```python
from build123d import *

# Parameters (mm, degrees)
SKETCH1_W           = 100
SKETCH1_H           = 200
BOSS_EXTRUDE1_DEPTH = 2.5
SKETCH2_W           = 200
SKETCH2_H           = 70
BOSS_EXTRUDE2_DEPTH = 2.5
SKETCH3_R           = 8
CUT_EXTRUDE1_DEPTH  = 5
SKETCH4_W           = 105
SKETCH4_H           = 70
BOSS_EXTRUDE3_DEPTH = 10
SKETCH5_W           = 105
SKETCH5_H           = 70
BOSS_EXTRUDE4_DEPTH = 5
SKETCH6_W           = 100
SKETCH6_H           = 30
CUT_EXTRUDE2_DEPTH  = 167.37683132
SKETCH7_R           = 4
CUT_EXTRUDE5_DEPTH  = 232.381719243
SKETCH7_5_R         = 3
SKETCH7_5_R_2       = 8
CUT_EXTRUDE6_DEPTH  = 5
SKETCH8_R           = 8
CUT_EXTRUDE7_DEPTH  = 6
SKETCH9_W           = 105
SKETCH9_H           = 175
CUT_EXTRUDE8_DEPTH  = 15


with BuildPart() as part:
    # Sketch1 → Boss-Extrude1 (new, symmetric)
    with BuildSketch(Plane(origin=(0, 0, 0), x_dir=(1, 0, 0), z_dir=(0, 1, 0))):
        Rectangle(SKETCH1_W, SKETCH1_H)
    extrude(amount=BOSS_EXTRUDE1_DEPTH, both=True)

    # Sketch2 → Boss-Extrude2 (add, symmetric)
    with BuildSketch(Plane.ZY.offset(50)):
        with Locations((0, 32.5)):
            Rectangle(SKETCH2_W, SKETCH2_H)
    boss_extrude2 = extrude(amount=BOSS_EXTRUDE2_DEPTH, both=True)

    # Sketch3 → Cut-Extrude1 (cut)
    with BuildSketch(Plane.ZY.offset(52.5)):
        with Locations((-80, 25)):
            Circle(SKETCH3_R)
        with Locations((80, 25)):
            Circle(SKETCH3_R)
    cut_extrude1 = extrude(amount=-CUT_EXTRUDE1_DEPTH, mode=Mode.SUBTRACT)

    # Mirror1: Boss-Extrude2, Cut-Extrude1 across plane
    add(boss_extrude2.mirror(Plane(origin=(0, 0, 0), x_dir=(0, 0, 1), z_dir=(1, 0, 0))))
    add(cut_extrude1.mirror(Plane(origin=(0, 0, 0), x_dir=(0, 0, 1), z_dir=(1, 0, 0))), mode=Mode.SUBTRACT)

    # Sketch4 → Boss-Extrude3 (add)
    with BuildSketch(Plane(origin=(0, 0, -100), x_dir=(-1, 0, 0), z_dir=(0, 0, -1))):
        with Locations((0, 32.5)):
            Rectangle(SKETCH4_W, SKETCH4_H)
    extrude(amount=BOSS_EXTRUDE3_DEPTH)

    # Sketch5 → Boss-Extrude4 (add)
    with BuildSketch(Plane.XY.offset(100)):
        with Locations((0, 32.5)):
            Rectangle(SKETCH5_W, SKETCH5_H)
    extrude(amount=BOSS_EXTRUDE4_DEPTH)

    # Sketch6 → Cut-Extrude2 (cut, through all)
    with BuildSketch(Plane.ZY.offset(52.5)):
        with Locations((0, 25)):
            Rectangle(SKETCH6_W, SKETCH6_H)
    extrude(amount=-CUT_EXTRUDE2_DEPTH, mode=Mode.SUBTRACT)

    # Sketch7 → Cut-Extrude5 (cut, through all)
    with BuildSketch(Plane(origin=(0, 0, 105), x_dir=(-1, 0, 0), z_dir=(0, 0, -1))):
        with Locations(Location((35, 40.5, 0), (0, 0, 180))):
            Circle(SKETCH7_R)
        with Locations(Location((-35, 40.5, 0), (0, 0, 180))):
            Circle(SKETCH7_R)
    extrude(amount=CUT_EXTRUDE5_DEPTH, mode=Mode.SUBTRACT)

    # Sketch7<5> → Cut-Extrude6 (cut)
    with BuildSketch(Plane(origin=(0, 0, 105), x_dir=(-1, 0, 0), z_dir=(0, 0, -1))):
        with Locations(Location((15.5, 56, 0), (0, 0, 180))):
            Circle(SKETCH7_5_R)
        with Locations(Location((-15.5, 56, 0), (0, 0, 180))):
            Circle(SKETCH7_5_R)
        with Locations(Location((15.5, 25, 0), (0, 0, 180))):
            Circle(SKETCH7_5_R)
        with Locations(Location((-15.5, 25, 0), (0, 0, 180))):
            Circle(SKETCH7_5_R)
        with Locations(Location((0, 40.5, 0), (0, 0, 180))):
            Circle(SKETCH7_5_R_2)
    extrude(amount=CUT_EXTRUDE6_DEPTH, mode=Mode.SUBTRACT)

    # Sketch8 → Cut-Extrude7 (cut)
    with BuildSketch(Plane(origin=(0, 0, -100), x_dir=(-1, 0, 0), z_dir=(0, 0, -1))):
        with Locations(Location((0, 40.5, 0), (0, 0, 180))):
            Circle(SKETCH8_R)
    extrude(amount=CUT_EXTRUDE7_DEPTH, mode=Mode.SUBTRACT)

    # Sketch9 → Cut-Extrude8 (cut)
    with BuildSketch(Plane(origin=(0, 67.5, 0), x_dir=(1, 0, 0), z_dir=(0, 1, 0))):
        with Locations((0, 22.5)):
            Rectangle(SKETCH9_W, SKETCH9_H)
    extrude(amount=-CUT_EXTRUDE8_DEPTH, mode=Mode.SUBTRACT)


solid = part.part
```
Input: part model. Units: mm. Frame: model coordinates. A direction names the side the tool comes from. Round coordinates to 2 decimals unless told otherwise and drop trailing zeros. Write each loop counter-clockwise with the first axis right and the second up, starting at its lowest first coordinate (ties: lowest second). Pieces come first, ordered by that corner, then holes. Notation, with made-up numbers: (-38.75, 77) - (-15.75, 77) arc R26 cw to (-15.75, 96) - close; hole circle Ø6 at (-35, 69). An arc over 180 degrees is marked (long way). Write item = value, one per line.
(1) Pull-direction query (Y, two-part tool) for faces 6 (the flat face through (-1, -2.5, -4)), 7 (the flat face through (47.5, 43, -1)), 8 (the cylindrical face through (-50, 30.4, -85.9)); classes: +Y half, -Y half, draft (parallel to the pull), parting line (faces both ways), or undercut.
Geometry check:
face_6 = -Y half
face_7 = draft
face_8 = undercut
(2) Material intervals for probe 1 along X at (y, z) = (25, 103); probe 2 along Y at (x, z) = (15, 103); probe 3 along X at (y, z) = (40.5, 102.9), sorted ascending.
Geometry check:
probe_1 = -52.5 to -18.5, -12.5 to 12.5, 18.5 to 52.5
probe_2 = -2.5 to 22.04, 27.96 to 53.04, 58.96 to 67.5
probe_3 = -52.5 to -39, -31 to -8, 8 to 31, 39 to 52.5
(3) Access query for faces 1 (the flat face through (-1, 2.5, -1)), 2 (the flat face through (50, 40, -1)), 3 (the flat face through (0, 40, -106)), 4 (the cylindrical face through (-35.521, 36.534, -104.93)), 5 (the flat face through (-50, 60, 65)). Directions: +Z, -Z, +X, -X, +Y, -Y. A direction counts if a zero-diameter tool reaches every point of the face in a straight line with its end or side. Return the directions, or none.
Geometry check:
face_1 = +Y
face_2 = +X, -X
face_3 = +Z
face_4 = +Z, -Z
face_5 = -Z, +X, -X, +Y
(4) Section query D-D on y = 30.5. State how many separate pieces and enclosed holes the cut face has, then the cut area to 3 significant figures.
Geometry check:
separate_pieces = 6
enclosed_holes = 0
area = 2,340 mm^2
(5) Section query A-A on z = 23. Output: boundary loops of the cut face in (x, y).
Geometry check:
outline = (-52.5, -2.5) - (52.5, -2.5) - (52.5, 10) - (47.5, 10) - (47.5, 2.5) - (-47.5, 2.5) - (-47.5, 10) - (-52.5, 10) - close; (-52.5, 40) - (-47.5, 40) - (-47.5, 52.5) - (-52.5, 52.5) - close; (47.5, 40) - (52.5, 40) - (52.5, 52.5) - (47.5, 52.5) - close
(6) Contact query for flat-ended pins moving along their axis: pin 1 Ø14.5 at (y, z) = (25, -80) entering from +X; pin 2 Ø5 at (x, y) = (2.5, 37) entering from +Z; pin 3 Ø5.5 at (x, y) = (-50, 60.5) entering from -Z; pin 4 Ø1.5 at (x, z) = (-50.5, 15) entering from +Y. Output: stop coordinate, or through.
Geometry check:
pin_1 = through
pin_2 = -106
pin_3 = 65
pin_4 = 52.5
(7) Section query B-B on x = -35. Output: boundary loops of the cut face in (y, z).
Geometry check:
outline = (-2.5, -110) - (36.5, -110) - (36.5, -100) - (2.5, -100) - (2.5, 100) - (36.5, 100) - (36.5, 105) - (-2.5, 105) - close; (44.5, -110) - (52.5, -110) - (52.5, -100) - (44.5, -100) - close; (44.5, 100) - (67.5, 100) - (67.5, 105) - (44.5, 105) - close
(8) Section query C-C on y = 63. Output: boundary loops of the cut face in (x, z), then the cut area to 3 significant figures.
Geometry check:
outline = (-52.5, 65) - (-47.5, 65) - (-47.5, 100) - (47.5, 100) - (47.5, 65) - (52.5, 65) - (52.5, 105) - (-52.5, 105) - close
area = 875 mm^2
